Autodesk Fusion 360 part; units mm, degrees
sketch "Sketch1" plane through (0, 0, 0) normal (0, 0, 1) x (1, 0, 0)
  line L0 (0, 0) -> (8, 0)
  line L1 (8, 0) -> (38, 0) construction
  line L2 (38, 0) -> (38, 40.25) construction
  circle A0 centre (38, 40.25) radius 1.3
  line L3 (41.5, 36.75) -> (34.5, 36.75)
  line L4 (34.5, 36.75) -> (34.5, 43.75)
  line L5 (34.5, 43.75) -> (41.5, 43.75)
  line L6 (41.5, 43.75) -> (41.5, 36.75)
  line L7 (41.5, 36.75) -> (34.5, 43.75) construction
  line L8 (34.5, 36.75) -> (41.5, 43.75) construction
  line L9 (8, 0) -> (34.5, 36.75)
  line L10 (38, 0) -> (68, 0) construction
  line L11 (68, 0) -> (76, 0)
  line L12 (68, 0) -> (41.5, 36.75)
  line L13 (76, 0) -> (76, -3.5)
  line L14 (76, -3.5) -> (68, -3.5)
  line L15 (0, 0) -> (0, -3.5)
  line L16 (0, -3.5) -> (8, -3.5)
  line L17 (11.2549, 4.5139) -> (14.0938, 2.4668) construction
  line L18 (8, -3.5) -> (9.7912, -3.5)
  line L19 (14.0938, 2.4668) -> (38, 35.6197)
  line L20 (65.1473, 3.9562) -> (62.3083, 1.9091) construction
  line L21 (62.3083, 1.9091) -> (38, 35.6197)
  line L22 (68, -3.5) -> (66.2088, -3.5)
  line L23 (8, 0) -> (12.315, 0)
  line L24 (68, 0) -> (63.685, 0)
  line L25 (14.0938, 2.4668) -> (12.315, 0)
  line L26 (12.315, 0) -> (12.315, -3.5)
  line L27 (12.315, -3.5) -> (9.7912, -3.5)
  line L28 (62.3083, 1.9091) -> (63.685, 0)
  line L29 (63.685, 0) -> (63.685, -3.5)
  line L30 (66.2088, -3.5) -> (63.685, -3.5)
  point P0 (38, 40.25)
  dimension "d1" = 8
  dimension "d2" = 30
  dimension "d3" = 40.25
  dimension "d4" = 2.6
  dimension "d5" = 7
  dimension "d6" = 7
  dimension "d7" = 30
  dimension "d8" = 8
  dimension "d9" = 3.5
  dimension "d10" = 3.5
extrude "Extrude1" add sketch "Sketch1" along normal blind 4 contours L3 L9 L12 L19 L21 L23 L24 L25 L28 | L3 L4 L5 L6 makes body 1
extrude "Extrude2" add sketch "Sketch1" along normal blind 6 separate body contours L0 L15 L16 L18 L23 L26 L27 | L11 L13 L14 L22 L24 L29 L30 makes body 2 at (67.79, 0, 2) makes body 3 at (4.105, 0, 2)
extrude "Extrude3" add sketch "Sketch1" against normal blind 2 contours L0 L15 L16 L18 L23 L26 L27 | L11 L13 L14 L22 L24 L29 L30 bodies 1 2 3
sketch "Sketch2" plane through (0, 0, 0) normal (0, 1, 0) x (-1, 0, 0)
  line L0 (-12.315, 4) -> (-8, 4)
  line L1 (-8, 4) -> (-8, 0)
  line L2 (-8, 0) -> (-12.315, 0)
  line L3 (-12.315, -2) -> (0, -2)
  line L4 (0, -2) -> (0, 6)
  line L5 (0, 6) -> (-12.315, 6)
  line L6 (-8.0111, 1.6089) -> (0, 2) construction
  line L7 (-4, 6) -> (-4, -2) construction
  circle A0 centre (-4, 2) radius 1.875
  line L8 (-12.315, 0) -> (-12.315, -2)
  line L9 (-12.315, 6) -> (-12.315, 4)
  dimension "d19" = 4
  dimension "d20" = 3.75
extrude "Extrude4" cut sketch "Sketch2" against normal blind 3.5 contours A0 bodies 1
sketch "Sketch3" plane through (0, 0, 0) normal (0, 1, 0) x (-1, 0, 0)
  line L0 (-68, 4) -> (-63.685, 4)
  line L1 (-63.685, 4) -> (-63.685, 6)
  line L2 (-63.685, 6) -> (-76, 6)
  line L3 (-76, 6) -> (-76, -2)
  line L4 (-76, -2) -> (-63.685, -2)
  line L5 (-63.685, -2) -> (-63.685, 0)
  line L6 (-63.685, 0) -> (-68, 0)
  line L7 (-68, 0) -> (-68, 4)
  line L8 (-76, 2) -> (-68, 2) construction
  line L9 (-72, 6) -> (-72, -2) construction
  circle A0 centre (-72, 2) radius 1.875
  dimension "d23" = 4
  dimension "d24" = 3.75
extrude "Extrude5" cut sketch "Sketch3" against normal blind 3.5 contours A0 bodies 1
fillet "Fillet1" radius 1 2 edges at (41.5, 36.75, 2) (34.5, 36.75, 2) on bodies 1
fillet "Fillet2" radius 1 3 edges at (68, 0, 2) (65.8425, 0, 0) (65.8425, 0, 4) on bodies 1
fillet "Fillet3" radius 1 3 edges at (8, 0, 2) (10.1575, 0, 4) (10.1575, 0, 0) on bodies 1
fillet "Fillet4" radius 1 1 edges at (38, 35.6197, 2) on bodies 1
Model file for the job. Use its own axes, mm. A direction names the side the tool comes from. Coordinates: 2 decimals unless noted, no trailing zeros. Order: outer loops, then holes, each group sorted by start corner. A loop starts at its lowest first (then second) coordinate and runs counter-clockwise, first axis right, second up. Notation, with made-up numbers: (24.5, 37.5) -> (49.5, 37.5) arc R25 ccw to (49.5, 75.5) -> close; hole circle Ø9 at (-30, 53). An arc over 180 degrees is marked (long way). Answer as a JSON object with one key per item and string values. Group by question number.
1) Drill centre lines: L1, parallel to Z at x = 72, y = -1 (3 decimals); L2, parallel to Y at x = 38, z = 2.7; L3, parallel to Y at x = 10, z = 5.75. Where is each one in solid material? Low to high.
2) Which spindle directions (+Z, -Z, +X, -X, +Y, -Y) get a long thin tool onto all of the face, cutting with end or side? Do faces 5 (the face through (73.38, -1.73, 3.27)), 6 (the face through (34.5, 40, 2)), 7 (the face through (63.685, -2, 2)). Say none if no direction does.
3) Cut at D-D, the plane x = 10. Write the cut outline in (y, z), then the cut area to 3 significant figures.
4) Flat gauge pins, fed straight in: pin 1 (2 mm diameter, centred on y = 26.5, z = 1, fed in from -X); pin 2 (3 mm diameter, centred on x = 9, z = -0.5, fed in from +Y); pin 3 (3 mm diameter, centred on y = 5.5, z = 3.5, fed in from -X). Where does each tip first touch, or does it go through?
5) Cut at A-A, the plane y = 40.25. Write the cut outline in (x, z), then the cut area to 3 significant figures.
6) Pull direction Z, two halves, no side cores. Call faces 1 (the face through (6, -2, 6)), 2 (the face through (70, -2, -2)), 3 (the face through (41.5, 40, 2)), 4 (the face through (5.49, -1.73, 0.86)): +Z half, -Z half, draft (parallel to the pull), parting line (faces both ways), or undercut.
7) Cut at C-C, the plane x = 38. Write the cut outline in (y, z).
8) Cut at B-B, the plane z = 2. Count the separate pieces of the cut face and the enclosed holes in it, then the cut area to 3 significant figures.
Check values:
{
 "1": {"L1": "z = -2 to 0.125, 3.875 to 6", "L2": "y = 34.91 to 38.95, 41.55 to 43.75", "L3": "y = -3.5 to 0"},
 "2": {"face 5": "+Y, -Y", "face 6": "+Z, -Z, -X, +Y", "face 7": "+Z, -Z, -Y"},
 "3": {"outline": "(-3.5, -2) -> (0, -2) -> (0, -1) arc R1 cw to (1, 0) -> (2.77, 0) -> (2.77, 4) -> (1, 4) arc R1 cw to (0, 5) -> (0, 6) -> (-3.5, 6) -> close", "area": "39.5 mm²"},
 "4": {"pin 1": "stops at x = 26.39", "pin 2": "stops at y = 3.35", "pin 3": "stops at x = 10.88"},
 "5": {"outline": "(34.5, 0) -> (36.7, 0) -> (36.7, 4) -> (34.5, 4) -> close; (39.3, 0) -> (41.5, 0) -> (41.5, 4) -> (39.3, 4) -> close", "area": "17.6 mm²"},
 "6": {"face 1": "+Z half", "face 2": "-Z half", "face 3": "draft", "face 4": "undercut"},
 "7": {"outline": "(34.91, 0) -> (38.95, 0) -> (38.95, 4) -> (34.91, 4) -> close; (41.55, 0) -> (43.75, 0) -> (43.75, 4) -> (41.55, 4) -> close"},
 "8": {"separate pieces": "3", "enclosed holes": "1", "area": "420 mm²"}
}
